Autodesk Inventor part; units mm, degrees
ref_plane "YZ Plane" through (0, 0, 0) normal (1, 0, 0) x (0, 1, 0)
ref_plane "XZ Plane" through (0, 0, 0) normal (0, 1, 0) x (-1, 0, 0)
ref_plane "XY Plane" through (0, 0, 0) normal (0, 0, 1) x (1, 0, 0)
sketch "Sketch1" plane through (0, 0, 0) normal (0, 0, 1) x (1, 0, 0)
  line L0 (0, 0) -> (5, 0)
  line L1 (5, 0) -> (5, 44)
  line L2 (5, 44) -> (0, 44)
  line L3 (0, 44) -> (0, 0)
  line L4 (5, 6) -> (8, 6)
  line L5 (8, 6) -> (8, 16)
  line L6 (8, 16) -> (5, 16)
  line L7 (5, 16) -> (5, 6)
  line L8 (5, 22) -> (0, 22) construction
  line L9 (2.5, 22) -> (2.5, 0) construction
  line L10 (0, 6) -> (-3, 6)
  line L11 (-3, 6) -> (-3, 16)
  line L12 (-3, 16) -> (0, 16)
  line L13 (5, 38) -> (8, 38)
  line L14 (8, 38) -> (8, 28)
  line L15 (8, 28) -> (5, 28)
  line L16 (-3, 28) -> (0, 28)
  line L17 (-3, 38) -> (-3, 28)
  line L18 (0, 38) -> (-3, 38)
  point P0 (6.5, 6)
  point P1 (-1.5, 6)
  point P2 (6.5, 38)
  point P3 (-1.5, 38)
  dimension "d0" = 5
  dimension "d1" = 44
  dimension "d2" = 3
  dimension "d3" = 6
  dimension "d4" = 10
extrude "Extrusion1" add sketch "Sketch1" along normal blind 3
properties part number "columna2"
Design review of the part built by this model. Coordinates are the model's own, in mm. A direction names the side the tool comes from. Round coordinates to 2 decimals unless told otherwise and drop trailing zeros. Write each loop counter-clockwise with the first axis right and the second up, starting at its lowest first coordinate (ties: lowest second). Pieces come first, ordered by that corner, then holes. Notation, with made-up numbers: (26.25, 76) - (41.25, 76) arc R27 cw to (41.25, 111) - close; hole circle Ø1 at (45.25, 73). An arc over 180 degrees is marked (long way). Return JSON: item names as keys, results as strings. Group by question number.
Item 1: We need section B-B on z = 1.3. Write out the cut boundary in (x, y).
Item 2: We need section A-A on x = -0.5. Write out the cut boundary in (y, z), and give its area (3 significant figures).
Item 3: For probe 1 along Y at (x, z) = (5.5, 1.8); probe 2 along X at (y, z) = (5.5, 0.2), list the stretches that pass through material, from the lowest coordinate up. Write a range as [from, to].
Item 4: The part is to be moulded in two halves that separate along Y. For faces 1 (the face through (5, 22, 1)), 2 (the face through (-3, 11, 1)), 3 (the face through (7, 28, 1)), 4 (the face through (2, 0, 1)), say which applies: pulls with the +Y half, pulls with the -Y half, needs draft (parallel to the pull), parting line crosses it, or undercut.
Item 5: We need section C-C on y = 4. Write out the cut boundary in (x, z).
Item 6: Machinability: for faces 5 (the face through (6, 6, 1)), 6 (the face through (7, 16, 1)), 7 (the face through (-1, 6, 1)), 8 (the face through (-1, 38, 1)), 9 (the face through (-2, 16, 1)), which of the approach directions +Z, -Z, +X, -X, +Y, -Y give a long, thin tool a straight path to every point of the face, cutting with its end or side? Answer none if there is none.
Item 7: Insertion check: P1, Ø0.9, axis at x = 7, z = 2, coming from the -Y side; P2, Ø1.5, axis at y = 3, z = 1, coming from the -X side; P3, Ø1.5, axis at y = 19.5, z = 1.5, coming from the +X side. Each pin has a flat end and moves straight along its axis. Give the tip position at first contact, or say it passes through.
Model answer:
{
 "1": {"outline": "(-3, 6) - (0, 6) - (0, 0) - (5, 0) - (5, 6) - (8, 6) - (8, 16) - (5, 16) - (5, 28) - (8, 28) - (8, 38) - (5, 38) - (5, 44) - (0, 44) - (0, 38) - (-3, 38) - (-3, 28) - (0, 28) - (0, 16) - (-3, 16) - close"},
 "2": {"outline": "(6, 0) - (16, 0) - (16, 3) - (6, 3) - close; (28, 0) - (38, 0) - (38, 3) - (28, 3) - close", "area": "60.0 mm²"},
 "3": {"probe 1": "y = [6, 16], [28, 38]", "probe 2": "x = [0, 5]"},
 "4": {"face 1": "undercut", "face 2": "needs draft", "face 3": "undercut", "face 4": "pulls with the -Y half"},
 "5": {"outline": "(0, 0) - (5, 0) - (5, 3) - (0, 3) - close"},
 "6": {"face 5": "+Z, -Z, +X, -Y", "face 6": "+Z, -Z, +X", "face 7": "+Z, -Z, -X, -Y", "face 8": "+Z, -Z, -X, +Y", "face 9": "+Z, -Z, -X"},
 "7": {"P1": "stops at y = 6", "P2": "stops at x = 0", "P3": "stops at x = 5"}
}
